Geometry check sheet. Reference: the model listing, model coordinates, mm. Face numbers are marked on the shaded views. A direction names the side the tool comes from. Coordinates: 2 decimals unless noted, no trailing zeros. Loops run counter-clockwise (first coordinate to the right, second up) from the corner with the lowest first, then second, coordinate; pieces in that order, holes last.
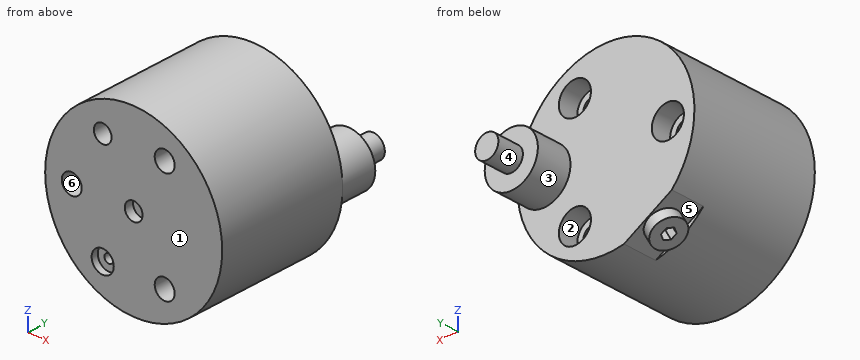
from build123d import *

# Parameters (mm, degrees)
SKETCH1_R          = 40
EXTRUDE1_DEPTH     = 59
SKETCH11_R         = 12
EXTRUDE2_DEPTH     = 16
SKETCH12_R         = 5.25
EXTRUDE3_DEPTH     = 12
HOLE1_D            = 9
HOLE1_DEPTH        = 59.001
HOLE1_CBORE_D      = 14.5
HOLE1_CBORE_DEPTH  = 9
CIRPATTERN1_COUNT  = 3
SKETCH5_R          = 4
CUT_EXTRUDE1_DEPTH = 4
SKETCH13_R         = 4
CUT_EXTRUDE5_DEPTH = 10
SKETCH6_R          = 5
CUT_EXTRUDE2_DEPTH = 3
SKETCH7_R          = 2
CUT_EXTRUDE3_DEPTH = 48.5
CUT_EXTRUDE6_DEPTH = 15.5
SKETCH8_W          = 15
SKETCH8_H          = 4.283
CUT_EXTRUDE4_DEPTH = 5


with BuildPart() as part:
    # Sketch1 → Extrude1 (new body)
    with BuildSketch(Plane(origin=(0, 0, 0), x_dir=(1, 0, 0), z_dir=(0, 1, 0))):
        with Locations(Location((0, 0, 0), (0, 0, 270))):  # turned: the seam where the file's is
            Circle(SKETCH1_R)
    extrude(amount=EXTRUDE1_DEPTH)

    # Sketch11 → Extrude2 (add)
    with BuildSketch(Plane(origin=(0, 59, 0), x_dir=(1, 0, 0), z_dir=(0, 1, 0))):
        with Locations((28, 0)):
            Circle(SKETCH11_R)
    extrude(amount=EXTRUDE2_DEPTH)

    # Sketch12 → Extrude3 (add)
    with BuildSketch(Plane(origin=(0, 75, 0), x_dir=(1, 0, 0), z_dir=(0, 1, 0))):
        with Locations(Location((28, 0, 0), (0, 0, 270))):  # turned: the seam where the file's is
            Circle(SKETCH12_R)
    extrude(amount=EXTRUDE3_DEPTH)

    # Hole1
    with Locations(Plane(origin=(0, 59, 0), x_dir=(-1, 0, 0), z_dir=(0, 1, 0))):
        with Locations((28, 0)):
            hole1 = CounterBoreHole(HOLE1_D / 2, HOLE1_CBORE_D / 2, HOLE1_CBORE_DEPTH, depth=HOLE1_DEPTH)

    # CirPattern1: Hole1 ×3 about axis
    cirpattern1_axis = Axis((0, 0, 0), (0, 1, 0))
    for i in range(1, CIRPATTERN1_COUNT):
        add(hole1.rotate(cirpattern1_axis, i * 360 / CIRPATTERN1_COUNT), mode=Mode.SUBTRACT)

    # Sketch5 → Cut-Extrude1 (cut)
    with BuildSketch(Plane.XZ):
        with Locations(Location((0, 0, 0), (0, 0, 270))):  # turned: the seam where the file's is
            Circle(SKETCH5_R)
    extrude(amount=-CUT_EXTRUDE1_DEPTH, mode=Mode.SUBTRACT)

    # Sketch13 → Cut-Extrude5 (cut)
    with BuildSketch(Plane.XZ):
        with Locations(Location((-14, 24.248711306, 0), (0, 0, 270))):  # turned: the seam where the file's is
            Circle(SKETCH13_R)
    extrude(amount=-CUT_EXTRUDE5_DEPTH, mode=Mode.SUBTRACT)

    # Sketch6 → Cut-Extrude2 (cut)
    with BuildSketch(Plane.XZ):
        with Locations(Location((-14, -24.248711306, 0), (0, 0, 270))):  # turned: the seam where the file's is
            Circle(SKETCH6_R)
    extrude(amount=-CUT_EXTRUDE2_DEPTH, mode=Mode.SUBTRACT)

    # Sketch7 → Cut-Extrude3 (cut)
    with BuildSketch(Plane.XZ.offset(-3)):
        with Locations(Location((-14, -24.248711306, 0), (0, 0, 270))):  # turned: the seam where the file's is
            Circle(SKETCH7_R)
    extrude(amount=-CUT_EXTRUDE3_DEPTH, mode=Mode.SUBTRACT)

    # Sketch14 → Cut-Extrude6 (cut)
    with BuildSketch(Plane(origin=(0, 59, 0), x_dir=(1, 0, 0), z_dir=(0, 1, 0))):
        with BuildLine():
            Line((-29.816653826, 26.663967345), (-8.183346174, 39.153963342))
            ThreePointArc((-8.183346174, 39.153963342), (-20, 34.641016151), (-29.816653826, 26.663967345))
        make_face()
    extrude(amount=-CUT_EXTRUDE6_DEPTH, mode=Mode.SUBTRACT)

    # Sketch8 → Cut-Revolve1 (revolve, cut)
    with BuildSketch(Plane(origin=(0, 0, 0), x_dir=(-0.5, 0, -0.866025404), z_dir=(0.866025404, 0, -0.5)), mode=Mode.PRIVATE) as cut_revolve1_sk:
        with Locations((30.5, 49.3585)):
            Rectangle(SKETCH8_W, SKETCH8_H)
    revolve(cut_revolve1_sk.sketch.rotate(Axis((-25.792798991, 51.5, -44.674438322), (0.5, 0, 0.866025404)), 270), axis=Axis((-25.792798991, 51.5, -44.674438322), (0.5, 0, 0.866025404)), mode=Mode.SUBTRACT)  # turned: the seam where the file's is

    # Sketch9 → Revolve2 (revolve)
    with BuildSketch(Plane(origin=(0, 0, 0), x_dir=(-0.5, 0, -0.866025404), z_dir=(0.866025404, 0, -0.5)), mode=Mode.PRIVATE) as revolve2_sk:
        Polygon((38, 44.5), (38, 47.217), (31.419, 47.217), (31, 47.636), (31, 51.5), (43, 51.5), (43, 44.5), align=None)
    revolve(revolve2_sk.sketch.rotate(Axis((-23.293952485, 51.5, -40.346309212), (0.5, 0, 0.866025404)), 270), axis=Axis((-23.293952485, 51.5, -40.346309212), (0.5, 0, 0.866025404)))  # turned: the seam where the file's is

    # Sketch10 → Cut-Extrude4 (cut)
    with BuildSketch(Plane(origin=(-21.5, 0, -37.239092363), x_dir=(-0.866025404, 0, 0.5), z_dir=(-0.5, 0, -0.866025404))):
        Polygon((2.886751346, 51.5), (1.443375673, 54), (-1.443375673, 54), (-2.886751346, 51.5), (-1.443375673, 49), (1.443375673, 49), align=None)
    extrude(amount=-CUT_EXTRUDE4_DEPTH, mode=Mode.SUBTRACT)


solid = part.part
1) Section check C-C on y = 72. Record the cut outline in (x, z), and give its area (3 significant figures).
Data:
outline: circle Ø24 at (28, 0)
area: 452 mm2
2) Depth check by flat-ended pin: pin 1 (5 mm diameter, centred on x = -14.5, z = -23, fed in from -Y); pin 2 (10 mm diameter, centred on x = -15.5, z = -34, fed in from +Y); pin 3 (4.5 mm diameter, centred on x = -30.5, z = -3, fed in from +Y); pin 4 (1 mm diameter, centred on x = -16.5, y = 60, fed in from -Z). Enter the tip coordinate at first touch or a pass-through.
Data:
pin 1: stops at y = 3
pin 2: stops at y = 59
pin 3: stops at y = 50
pin 4: passes through
3) Section check B-B on x = 0. Record the cut outline in (y, z), and give its area (3 significant figures).
Data:
outline: (0, -40) - (59, -40) - (59, 40) - (0, 40) - (0, 4) - (4, 4) - (4, -4) - (0, -4) - close
area: 4,690 mm2
4) Access from +Z, -Z, +X, -X, +Y, -Y to the whole of each face (thin tool, end or side, straight path). Record for the marked faces 4, 5 and 6.
Data:
face 4: +Y
face 5: none
face 6: +Y, -Y
5) Mould release check, pull along Z, two halves, no side actions. Record for the marked faces 1, 2 and 3: +Z half, -Z half, draft (parallel to the pull), parting line (faces both ways), or undercut.
Data:
face 1: draft
face 2: undercut
face 3: parting line
6) Section check A-A on z = -1.5. Record the cut outline in (x, y), and give its area (3 significant figures).
Data:
outline: (-39.97, 0) - (-32.24, 0) - (-32.24, 50) - (-35.09, 50) - (-35.09, 59) - (-39.97, 59) - close; (-23.76, 0) - (-3.71, 0) - (-3.71, 4) - (3.71, 4) - (3.71, 0) - (39.97, 0) - (39.97, 59) - (39.91, 59) - (39.91, 75) - (33.03, 75) - (33.03, 87) - (22.97, 87) - (22.97, 75) - (16.09, 75) - (16.09, 59) - (-20.91, 59) - (-20.91, 50) - (-23.76, 50) - close
area: 4,640 mm2
7) Material ranges on probe 1 along X at (y, z) = (24, -24.5); probe 2 along Z at (x, y) = (14, 56); probe 3 along Y at (x, z) = (30.5, 11), recorded low to high.
Data:
probe 1: x = -31.62 to -15.98, -12.02 to 9.51, 18.49 to 31.62
probe 2: z = -37.47 to -31.5, -17 to 17, 31.5 to 37.47
probe 3: y = 0 to 75
8) Section check D-D on y = 40.5. Record the cut outline in (x, z), and give its area (3 significant figures).
Data:
outline: circle Ø80 at (0, 0); hole circle Ø9 at (-28, 0); hole circle Ø4 at (-14, -24.25); hole circle Ø9 at (14, -24.25); hole circle Ø9 at (14, 24.25)
area: 4,820 mm2
